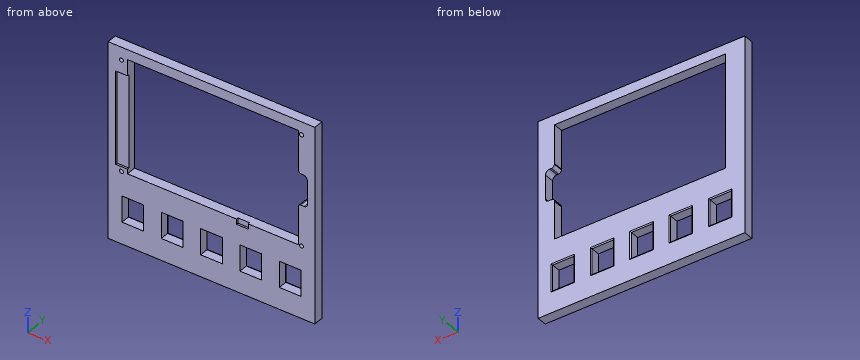
```python
from build123d import *

# Parameters (mm, degrees)
SKETCH1_W           = 105
SKETCH1_H           = 69
BOSS_EXTRUDE1_DEPTH = 5
SKETCH2_W           = 86.836
SKETCH2_H           = 57.499
CUT_EXTRUDE1_DEPTH  = 81.210380614
CUT_EXTRUDE2_DEPTH  = 1
SKETCH4_W           = 5
SKETCH4_H           = 2.165
SKETCH4_H_2         = 0.335
CUT_EXTRUDE3_DEPTH  = 1
CUT_EXTRUDE4_DEPTH  = 81.210380614
SKETCH9_R           = 1
CUT_EXTRUDE7_DEPTH  = 3
SKETCH7_W           = 105
SKETCH7_H           = 30
BOSS_EXTRUDE2_DEPTH = 5
SKETCH8_W           = 11
SKETCH8_H           = 13.2
CUT_EXTRUDE6_DEPTH  = 84.315664794
FILLET1_R           = 0.5
FILLET3_R           = 1


with BuildPart() as part:
    # Sketch1 → Boss-Extrude1 (new body)
    with BuildSketch(Plane(origin=(0, 0, 0), x_dir=(1, 0, 0), z_dir=(0, 1, 0))):
        Rectangle(SKETCH1_W, SKETCH1_H)
    extrude(amount=BOSS_EXTRUDE1_DEPTH)

    # Sketch2 → Cut-Extrude1 (cut, through all)
    with BuildSketch(Plane(origin=(17.072113262, 0, 5.103361153), x_dir=(-1, 0, 0), z_dir=(0, -1, 0))):
        with Locations((16.310113262, 4.341361153)):
            Rectangle(SKETCH2_W, SKETCH2_H)
    extrude(amount=-CUT_EXTRUDE1_DEPTH, mode=Mode.SUBTRACT)

    # Sketch3 → Cut-Extrude2 (cut)
    with BuildSketch(Plane(origin=(17.072113262, 0, 5.103361153), x_dir=(-1, 0, 0), z_dir=(0, -1, 0))):
        Polygon((59.822113262, 30.765861153), (54.524773562, 30.765861153), (54.524773562, -16.234138847), (59.822113262, -16.234138847), (65.822113262, -16.234138847), (65.822113262, 30.765861153), align=None)
    extrude(amount=-CUT_EXTRUDE2_DEPTH, mode=Mode.SUBTRACT)

    # Sketch4 → Cut-Extrude3 (cut)
    with BuildSketch(Plane(origin=(17.072113262, 0, 5.103361153), x_dir=(-1, 0, 0), z_dir=(0, -1, 0))):
        Polygon((-1.187888405, 35.255861153), (3.812111595, 35.255861153), (3.812111595, 33.090861153), (4.312111595, 33.090861153), (4.312111595, 35.755861153), (-1.687888405, 35.755861153), (-1.687888405, 33.090861153), (-1.187888405, 33.090861153), align=None)
        with Locations((1.312111595, 34.173361153)):
            Rectangle(SKETCH4_W, SKETCH4_H)
        Polygon((4.312111595, 33.090861153), (3.812111595, 33.090861153), (3.812111595, 32.755861153), (-1.187888405, 32.755861153), (-1.187888405, 33.090861153), (-1.687888405, 33.090861153), (-1.687888405, 32.255861153), (4.312111595, 32.255861153), align=None)
        with Locations((1.312111595, 32.923361153)):
            Rectangle(SKETCH4_W, SKETCH4_H_2)
    extrude(amount=-CUT_EXTRUDE3_DEPTH, mode=Mode.SUBTRACT)

    # Sketch5 → Cut-Extrude4 (cut, through all)
    with BuildSketch(Plane(origin=(17.072113262, 0, 5.103361153), x_dir=(-1, 0, 0), z_dir=(0, -1, 0))):
        with BuildLine():
            Line((-31.677886738, -0.896638847), (-31.677886738, 11.103361153))
            ThreePointArc((-31.677886738, 11.103361153), (-31.220399504, 12.207833039), (-30.115927617, 12.665320274))
            Line((-30.115927617, 12.665320274), (-28.350143546, 12.665320274))
            ThreePointArc((-28.350143546, 12.665320274), (-27.521232808, 13.008666344), (-27.177886738, 13.837577082))
            Line((-27.177886738, 13.837577082), (-18.865935491, 13.837577082))
            Line((-18.865935491, 13.837577082), (-18.865935491, -4.56597095))
            Line((-18.865935491, -4.56597095), (-27.177886738, -4.56597095))
            ThreePointArc((-27.177886738, -4.56597095), (-27.60841615, -3.526581006), (-28.647806094, -3.096051594))
            Line((-28.647806094, -3.096051594), (-29.478473991, -3.096051594))
            ThreePointArc((-29.478473991, -3.096051594), (-31.033693659, -2.451858515), (-31.677886738, -0.896638847))
        make_face()
    extrude(amount=-CUT_EXTRUDE4_DEPTH, mode=Mode.SUBTRACT)

    # Sketch9 → Cut-Extrude7 (cut)
    with BuildSketch(Plane(origin=(17.072113262, 0, 5.103361153), x_dir=(-1, 0, 0), z_dir=(0, -1, 0))):
        with Locations(Location((-28.677886738, 33.103361153, 0), (0, 0, 90))):
            Circle(SKETCH9_R)
        with Locations(Location((62.822113262, 33.103361153, 0), (0, 0, 90))):
            Circle(SKETCH9_R)
        with Locations(Location((-28.677886738, -22.896638847, 0), (0, 0, 90))):
            Circle(SKETCH9_R)
        with Locations(Location((62.822113262, -22.896638847, 0), (0, 0, 90))):
            Circle(SKETCH9_R)
    extrude(amount=-CUT_EXTRUDE7_DEPTH, mode=Mode.SUBTRACT)

    # Sketch7 → Boss-Extrude2 (add)
    with BuildSketch(Plane(origin=(0, 5, 0), x_dir=(1, 0, 0), z_dir=(0, 1, 0))):
        with Locations((0, 49.5)):
            Rectangle(SKETCH7_W, SKETCH7_H)
    extrude(amount=-BOSS_EXTRUDE2_DEPTH)

    # Sketch8 → Cut-Extrude6 (cut, through all)
    with BuildSketch(Plane(origin=(0, 5, 0), x_dir=(1, 0, 0), z_dir=(0, 1, 0))):
        with Locations((20, 46.886314888)):
            Rectangle(SKETCH8_W, SKETCH8_H)
        with Locations((40, 46.886314888)):
            Rectangle(SKETCH8_W, SKETCH8_H)
        with Locations((0, 46.886314888)):
            Rectangle(SKETCH8_W, SKETCH8_H)
        with Locations((-20, 46.886314888)):
            Rectangle(SKETCH8_W, SKETCH8_H)
        with Locations((-40, 46.886314888)):
            Rectangle(SKETCH8_W, SKETCH8_H)
    extrude(amount=-CUT_EXTRUDE6_DEPTH, mode=Mode.SUBTRACT)

    # Fillet1
    fillet1_edges = [part.edges().sort_by_distance(p)[0] for p in [
        (34.5, 5, -46.886314888),
        (40, 5, -40.286314888),
        (45.5, 5, -46.886314888),
        (40, 5, -53.486314888),
        (20, 5, -53.486314888),
        (14.5, 5, -46.886314888),
        (20, 5, -40.286314888),
        (25.5, 5, -46.886314888),
        (0, 5, -53.486314888),
        (-5.5, 5, -46.886314888),
        (0, 5, -40.286314888),
        (5.5, 5, -46.886314888),
        (-20, 5, -53.486314888),
        (-25.5, 5, -46.886314888),
        (-20, 5, -40.286314888),
        (-14.5, 5, -46.886314888),
        (-40, 5, -53.486314888),
        (-45.5, 5, -46.886314888),
        (-40, 5, -40.286314888),
        (-34.5, 5, -46.886314888),
    ]]
    fillet(fillet1_edges, radius=FILLET1_R)

    # Fillet3
    # the kernel refuses this fillet: 1 mm, written as the material it takes off along each edge
    with BuildSketch(Plane(origin=(44.18, -0.918898797, 9.669332102), x_dir=(0, 0, 1), z_dir=(0, 1, 0)), Plane(origin=(44.18, 5.918898797, -8.734215929), x_dir=(0, 0, -1), z_dir=(0, -1, 0))) as fillet3_piece_1:
        with BuildLine():
            CenterArc((0.367559519, 1), FILLET3_R, 248.434814985, 21.565185015)
            Line((0, 0.07), (-0.00735119, 0.0514))
            ThreePointArc((-0.00735119, 0.0514), (-0.02, 0.035), (-0.02, 0))
            Line((-0.02, 0), (0, -0.02))
            Line((0, -0.02), (0.367559519, -0.02))
            Line((0.367559519, -0.02), (0.367559519, 0))
        make_face()
    extrude(amount=6.837797595, mode=Mode.SUBTRACT)


solid = part.part
```
Design review of the part built by this model. Coordinates are the model's own, in mm. Coordinates: 2 decimals unless noted, no trailing zeros. Order: outer loops, then holes, each group sorted by start corner. A loop starts at its lowest first (then second) coordinate and runs counter-clockwise, first axis right, second up. Notation, with made-up numbers: M -9,-13 L 6,-13 A20 cw 6,4 Z; hole C 65,11 d11. An arc over 180 degrees is marked long. Answer as a JSON object with one key per item and string values. Group by question number.
1) Add section B-B, the plane x = 42. Write out the cut boundary in (y, z).
2) Wall thickness on L1, parallel to X at y = 1.95, z = 28; L2, parallel to Z at x = 2, y = 4.4; L3, parallel to X at y = 1.15, z = -41: over which ranges is each line inside the solid? List them lowest first.
3) For pin 1 (3 mm diameter, centred on x = -47, z = -2, fed in from -Y), flat-tipped, find the tip position at first contact; note if it passes through.
4) Add section C-C, the plane z = 0. Write out the cut boundary in (x, y), then the cut area to 3 significant figures.
5) Add section A-A, the plane z = -47. Count the separate pieces of the cut face and the enclosed holes in it, then the cut area to 3 significant figures.
Computed values:
{
 "1": {"outline": "M 0,-64.5 L 5,-64.5 L 5,-53.99 A0.5 ccw 4.5,-53.49 L 0,-53.49 Z; M 0,-40.29 L 4.5,-40.29 A0.5 ccw 5,-39.79 L 5,-27.99 L 0,-27.99 Z; M 0,29.51 L 5,29.51 L 5,34.5 L 0,34.5 Z"},
 "2": {"L1": "x = -52.5 to -46.75, -44.75 to -42.66, 44.18 to 44.75, 46.75 to 52.5", "L2": "z = -64.5 to -53.49, -40.29 to -27.99, 29.51 to 34.5", "L3": "x = -52.5 to -45.5, -34.5 to -25.5, -14.5 to -5.5, 5.5 to 14.5, 25.5 to 34.5, 45.5 to 52.5"},
 "3": {"pin 1": "stops at y = 1"},
 "4": {"outline": "M -52.5,0 L -48.75,0 L -48.75,1 L -42.66,1 L -42.66,5 L -52.5,5 Z; M 48.75,0 L 52.5,0 L 52.5,5 L 48.75,5 Z", "area": "61.9 mm^2"},
 "5": {"separate pieces": "6", "enclosed holes": "0", "area": "249 mm^2"}
}
